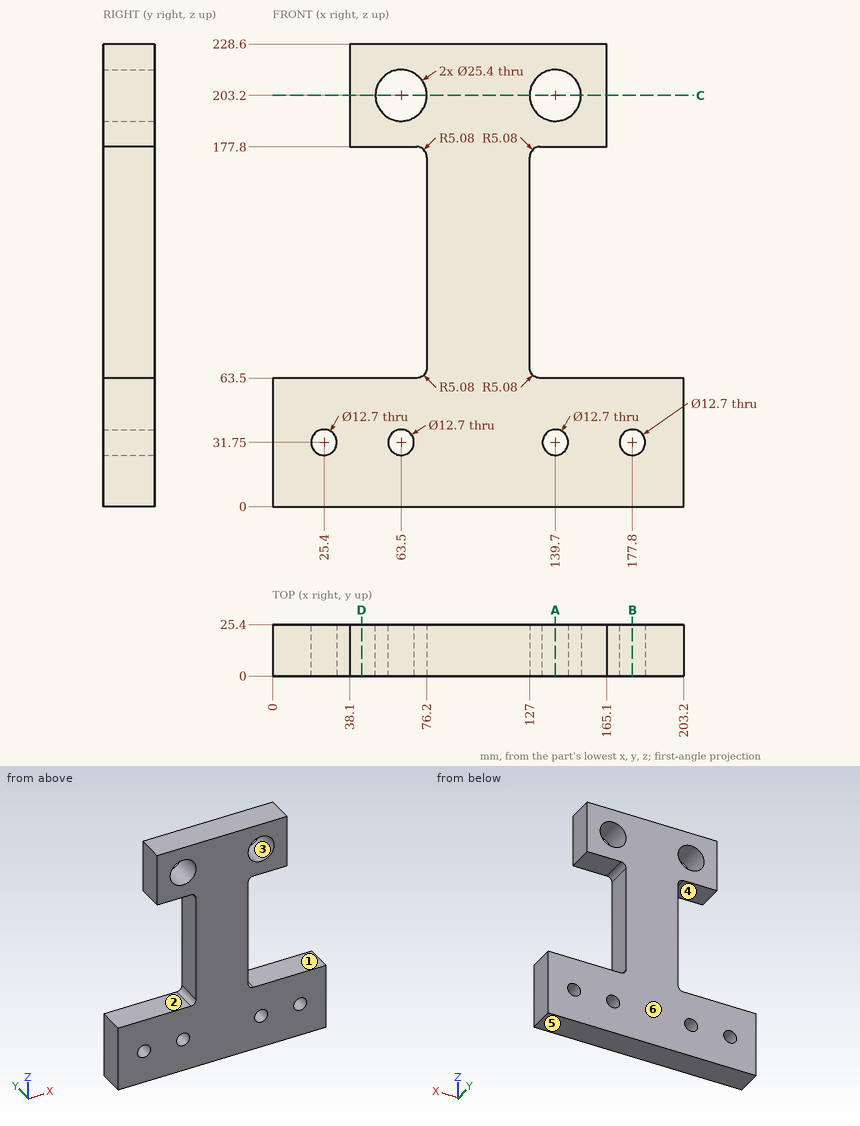
Answer from the drawing. Dimensions are ordinates in mm from the lowest x, y and z of the part. A direction names the side the tool comes from. Give positions to 0.01 mm unless a question says otherwise; leave off trailing zeros. Order: outer loops, then holes, each group sorted by start corner. A loop starts at its lowest first (then second) coordinate and runs counter-clockwise, first axis right, second up. Notation, with made-up numbers: (-7.5, 40.25) - (20.5, 40.25) arc R24 cw to (20.5, 65.25) - close; hole circle Ø7 at (80.25, 24.25). An arc over 180 degrees is marked (long way). One line per item, written item: value. Start each with the question number.
1. For a pull along Z with two mould halves and no side action, classify the marked faces 4, 5 and 6 as released by +Z, released by -Z, zero draft, split by the parting line, or undercut.
2. Section C-C, the plane z = 203.2 is taken. Write down the section's boundary in (x, y), then the cut area to 3 significant figures.
3. Section A-A, the plane x = 139.7 is taken. Write down the section's boundary in (y, z).
4. Consider line 1 (Z direction, x = 63, y = 12.5); line 2 (Z direction, x = 164.5, y = 14.25); line 3 (X direction, y = 11.25, z = 215). Determine where each line is inside the solid, lowest interval first.
5. Section B-B, the plane x = 177.8 is taken. Write down the section's boundary in (y, z), then the cut area to 3 significant figures.
6. Section D-D, the plane x = 44 is taken. Write down the section's boundary in (y, z).
7. Which of the six approach directions +Z, -Z, +X, -X, +Y, -Y give full straight-line access (tool end or side, diameter ignored) to the marked faces 1, 2 and 3?
8. Each of these flat-tipped pins is pushed along its axis until it touches: pin 1 Ø12.5 at (x, y) = (152.5, 10.5) entering from -Z; pin 2 Ø7.5 at (y, z) = (16.5, 196.5) entering from +X; pin 3 Ø10 at (x, z) = (139.7, 31.75) entering from +Y; pin 4 Ø3 at (y, z) = (8.5, 170.5) entering from +X. Where does it stop, or does it pass through?
Filled sheet:
1. face 4: undercut
1. face 5: released by -Z
1. face 6: zero draft
2. outline: (38.1, 0) - (50.8, 0) - (50.8, 25.4) - (38.1, 25.4) - close; (76.2, 0) - (127, 0) - (127, 25.4) - (76.2, 25.4) - close; (152.4, 0) - (165.1, 0) - (165.1, 25.4) - (152.4, 25.4) - close
2. area: 1,940 mm²
3. outline: (0, 0) - (25.4, 0) - (25.4, 25.4) - (0, 25.4) - close; (0, 38.1) - (25.4, 38.1) - (25.4, 63.5) - (0, 63.5) - close; (0, 177.8) - (25.4, 177.8) - (25.4, 190.5) - (0, 190.5) - close; (0, 215.9) - (25.4, 215.9) - (25.4, 228.6) - (0, 228.6) - close
4. line 1: 0 to 25.42, 38.08 to 63.5, 177.8 to 190.51, 215.89 to 228.6
4. line 2: 0 to 63.5, 177.8 to 228.6
4. line 3: 38.1 to 58.8, 68.2 to 135, 144.4 to 165.1
5. outline: (0, 0) - (25.4, 0) - (25.4, 25.4) - (0, 25.4) - close; (0, 38.1) - (25.4, 38.1) - (25.4, 63.5) - (0, 63.5) - close
5. area: 1,290 mm²
6. outline: (0, 0) - (25.4, 0) - (25.4, 63.5) - (0, 63.5) - close; (0, 177.8) - (25.4, 177.8) - (25.4, 228.6) - (0, 228.6) - close
7. face 1: +X, +Y, -Y
7. face 2: -X, +Y, -Y
7. face 3: +Y, -Y
8. pin 1: z = 0
8. pin 2: x = 165.1
8. pin 3: through
8. pin 4: x = 127
